Can you work these out from the model? Positions are in its coordinate system, mm. Face numbers are marked on the shaded views. A direction names the side the tool comes from. Round coordinates to 2 decimals unless told otherwise and drop trailing zeros. Order: outer loops, then holes, each group sorted by start corner. A loop starts at its lowest first (then second) coordinate and runs counter-clockwise, first axis right, second up.
Q1. If we section it at B-B (x = 0): Please give me the cut outline in (y, z), plus the area to 3 significant figures.
Q2. If we section it at C-C (y = -9): Count the separate pieces of the cut face and the enclosed holes in it, plus the area to 3 significant figures.
Q3. If I drill on line 1 (Z direction, x = -30, y = -14); line 2 (Y direction, x = 27.5, z = 11); line 3 (Z direction, x = -31, y = -1.75), over which ranges is the centre line in solid material (lowest first)?
Q4. For the marked faces 4, 5, 6 and 7, which set-ups out of +Z, -Z, +X, -X, +Y, -Y let a thin tool reach every point of the face, with its end or its side?
Q5. If we section it at A-A (z = 8): Please give me the cut outline in (x, y).
Q6. We'd pull the mould along X, two halves only. Please class the marked faces 1, 2 and 3: pulls with the +X half, pulls with the -X half, needs draft (parallel to the pull), parting line crosses it, or undercut.
Q7. Will these pins go through, and if not, where does the flat tip stop? P1, Ø3, axis at x = 26, y = -11, coming from the -Z side; P2, Ø1, axis at y = -17, z = 11.5, coming from the +X side; P3, Ø4, axis at x = 23, z = 10.5, coming from the -Y side; P4, Ø12, axis at x = -0.5, y = -18.5, coming from the +Z side.
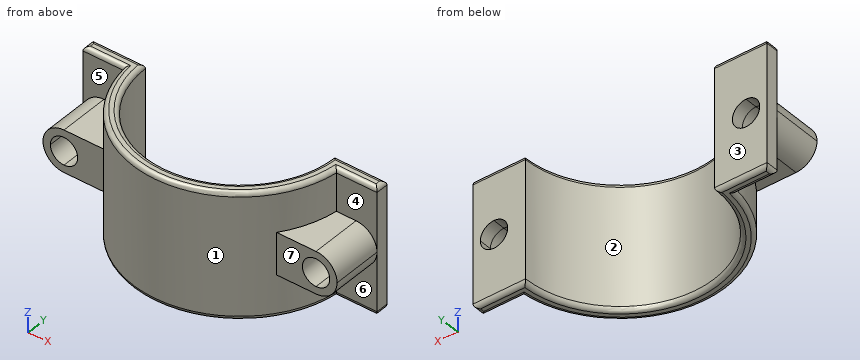
from build123d import *

# Parameters (mm, degrees)
BOSS_EXTRUDE1_DEPTH = 15
CUT_EXTRUDE1_DEPTH  = 45.229515196
FILLET1_R           = 1


with BuildPart() as part:
    # Sketch1 → Boss-Extrude1 (new, symmetric)
    with BuildSketch(Plane.XY):
        with BuildLine():
            Line((-35, 0), (-22.5, 0))
            ThreePointArc((-22.5, 0), (0, -22.5), (22.5, 0))
            Line((22.5, 0), (35, 0))
            Line((35, 0), (35, -3))
            Line((35, -3), (25.322914524, -3))
            ThreePointArc((25.322914524, -3), (0, -25.5), (-25.322914524, -3))
            Line((-25.322914524, -3), (-35, -3))
            Line((-35, -3), (-35, 0))
        make_face()
    extrude(amount=BOSS_EXTRUDE1_DEPTH, both=True)

    # Boss-Extrude2: read off the stored shape, not the designer's step
    # Boss-Extrude2: loft between two sections, ruled curve by curve
    boss_extrude2_from = [
        Edge.make_three_point_arc((30, -3, -5), (33.535533906, -3, -3.535533906), (35, -3, 0)),
        Edge.make_three_point_arc((35, -3, 0), (33.535533906, -3, 3.535533906), (30, -3, 5)),
        Edge.make_line((25.322914524, -3, 5), (30, -3, 5)),
        Edge.make_line((25.322914524, -3, -5), (30, -3, -5)),
        Edge.make_line((25.322914524, -3, -5), (25.322914524, -3, 5)),
    ]
    boss_extrude2_to = [
        Edge.make_three_point_arc((30, -15, -5), (33.535533906, -15, -3.535533906), (35, -15, 0)),
        Edge.make_three_point_arc((35, -15, 0), (33.535533906, -15, 3.535533906), (30, -15, 5)),
        Edge.make_line((20.621590627, -15, 5), (30, -15, 5)),
        Edge.make_line((20.621590627, -15, -5), (30, -15, -5)),
        Edge.make_line((20.621590627, -15, -5), (20.621590627, -15, 5)),
    ]
    boss_extrude2 = Solid(Shell([*[Face.make_surface_from_curves(boss_extrude2_from[k], boss_extrude2_to[k]) for k in range(5)], Face(Wire(boss_extrude2_from)), Face(Wire(boss_extrude2_to))]))
    add(boss_extrude2)

    # Sketch2_3 → Cut-Extrude1 (cut, symmetric)
    with BuildSketch(Plane.XZ.offset(3)):
        with BuildLine():
            ThreePointArc((33.25, 0), (32.298097039, 2.298097039), (30, 3.25))
            Line((30, 3.25), (30, -3.25))
            ThreePointArc((30, -3.25), (32.298097039, -2.298097039), (33.25, 0))
        make_face()
        with BuildLine():
            Line((30, -3.25), (30, 3.25))
            ThreePointArc((30, 3.25), (26.75, 0), (30, -3.25))
        make_face()
    cut_extrude1 = extrude(amount=CUT_EXTRUDE1_DEPTH, both=True, mode=Mode.SUBTRACT)

    # Mirror1: Boss-Extrude2, Cut-Extrude1 across plane
    add(boss_extrude2.mirror(Plane(origin=(0, 0, 0), x_dir=(0, 0, 1), z_dir=(1, 0, 0))))
    add(cut_extrude1.mirror(Plane(origin=(0, 0, 0), x_dir=(0, 0, 1), z_dir=(1, 0, 0))), mode=Mode.SUBTRACT)

    # Fillet1
    fillet1_edges = [part.edges().sort_by_distance(p)[0] for p in [
        (-30.161457262, -3, -15),
        (-35, -1.5, -15),
        (-28.75, 0, -15),
        (0, -22.5, -15),
        (-35, -1.5, 15),
        (-30.161457262, -3, 15),
        (0, -25.5, 15),
        (30.161457262, -3, 15),
        (35, -1.5, 15),
        (28.75, 0, 15),
        (0, -22.5, 15),
        (28.75, 0, -15),
        (-28.75, 0, 15),
        (35, -1.5, -15),
        (30.161457262, -3, -15),
        (0, -25.5, -15),
    ]]
    fillet(fillet1_edges, radius=FILLET1_R)


solid = part.part
Solution:
1. outline: (-25.5, -14) arc R1 ccw to (-24.5, -15) - (-23.5, -15) arc R1 ccw to (-22.5, -14) - (-22.5, 14) arc R1 ccw to (-23.5, 15) - (-24.5, 15) arc R1 ccw to (-25.5, 14) - close
1. area: 89.1 mm2
2. separate pieces: 2
2. enclosed holes: 2
2. area: 327 mm2
3. line 1: z = -5 to -3.25, 3.25 to 5
3. line 2: y = -3 to 0
3. line 3: z = -15 to -3.09, 3.09 to 15
4. face 4: +Z, +X, -Y
4. face 5: +Z, -X, -Y
4. face 6: -Z, +X, -Y
4. face 7: +Z, -Z, +X, -Y
5. outline: (-35, -3) - (-25.32, -3) arc R25.5 ccw to (25.32, -3) - (35, -3) - (35, 0) - (22.5, 0) arc R22.5 cw to (-22.5, 0) - (-35, 0) - close
6. face 1: parting line crosses it
6. face 2: undercut
6. face 3: needs draft
7. P1: stops at z = -5
7. P2: stops at x = 19.44
7. P3: stops at y = -14.47
7. P4: stops at z = 15
